The model under review builds one solid part; all positions refer to its coordinate system, in mm. Face numbers are marked on the shaded views. A direction names the side the tool comes from. Coordinates: 2 decimals unless noted, no trailing zeros. Loops run counter-clockwise (first coordinate to the right, second up) from the corner with the lowest first, then second, coordinate; pieces in that order, holes last. Notation, with made-up numbers: M 43,-27.75 L 86,-27.75 A21 cw 86,-1.75 Z; hole C -39,77.5 d1. An arc over 180 degrees is marked long. Use CSV: the item, a comma, the result in double quotes. Start each with the question number.
1. Add section A-A, the plane z = -19.5. Write out the cut boundary in (x, y), then the cut area to 3 significant figures.
2. Draft analysis for pull direction X (two halves, no side actions). For the marked faces 4, 5, 6 and 7, state which applies: +X half, -X half, draft (parallel to the pull), parting line (faces both ways), or undercut.
3. Add section B-B, the plane x = -1. Write out the cut boundary in (y, z).
4. Clearance check with flat-ended pins moving along their axes: P1, Ø1.4, axis at x = -9.48, z = -4.81, coming from the -Y side; P2, Ø7.5, axis at x = 0, z = 0, coming from the +Y side; P3, Ø4, axis at y = 7.5, z = -31, coming from the -X side; P4, Ø4, axis at x = 18.5, z = -14.5, coming from the -Y side. State where each tip first meets the part, or that it passes through.
5. For L1, parallel to X at y = 2.75, z = -12.5; L2, parallel to Z at x = 12.5, y = 5.5; L3, parallel to Y at x = -1, z = -40, list the stretches that pass through material, from the lowest coordinate up.
6. Add section D-D, the plane x = -20. Write out the cut boundary in (y, z).
7. Tool access review of the marked faces 1, 2 and 3: name each direction out of +Z, -Z, +X, -X, +Y, -Y from which nothing blocks a thin tool from reaching the whole face with its end or side.
8. Add section C-C, the plane x = 23. Write out the cut boundary in (y, z), then the cut area to 3 significant figures.
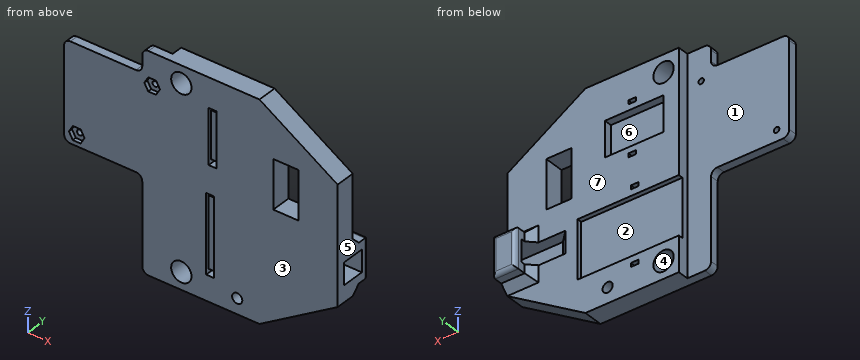
from build123d import *

# Parameters (mm, degrees)
SKETCH1_R               = 1.651
SKETCH1_R_2             = 3.302
SKETCH1_R_3             = 0.889
SKETCH1_W               = 8.2042
SKETCH1_H               = 15.748
BOSS_EXTRUDE1_DEPTH     = 6.35
SKETCH2_W               = 19.05
SKETCH2_H               = 11.43
CUT_EXTRUDE1_DEPTH      = 2.54
CUT_EXTRUDE2_DEPTH      = 83.161835082
CUT_EXTRUDE2_DEPTH_BACK = 83.161835082
SKETCH5_W               = 2.54
SKETCH5_H               = 1.27
SKETCH6_W               = 2.54
SKETCH6_H               = 15.24
CUT_EXTRUDE3_DEPTH      = 1.016
SKETCH7_W               = 40.64
SKETCH7_H               = 18.796
CUT_EXTRUDE4_DEPTH      = 1.524
CUT_EXTRUDE5_DEPTH      = 83.161835082
CUT_EXTRUDE5_DEPTH_BACK = 83.161835082
SKETCH8_W               = 2.54
SKETCH8_H               = 1.27
SKETCH10_W              = 2.54
SKETCH10_H              = 22.86
CUT_EXTRUDE6_DEPTH      = 1.016
SKETCH11_W              = 7.62
SKETCH11_H              = 12.7
BOSS_EXTRUDE2_DEPTH     = 6.35
SKETCH13_W              = 7.112
SKETCH13_H              = 7.493
CUT_EXTRUDE7_DEPTH      = 19.05
CHAMFER3_SIZE           = 2.54
FILLET1_R               = 1.27
CHAMFER4_SIZE           = 3.81
SKETCH14_W              = 33.125812981
SKETCH14_H              = 69.85
CUT_EXTRUDE8_DEPTH      = 3.556
FILLET2_R               = 2.032
CUT_EXTRUDE9_DEPTH      = 1.27


with BuildPart() as part:
    # Sketch1 → Boss-Extrude1 (new body)
    with BuildSketch(Plane(origin=(0, 0, 0), x_dir=(1, 0, 0), z_dir=(0, 1, 0))):
        Polygon((25.4, 64.262), (-12.7, 64.262), (-12.7, 33.782), (-38.1, 33.782), (-38.1, 2.032), (-12.7, 2.032), (-12.7, -5.588), (25.4, -5.588), (50.8, 10.287), (50.8, 48.387), align=None)
        with Locations(Location((18.161, 59.309, 0), (0, 0, 270))):
            Circle(SKETCH1_R, mode=Mode.SUBTRACT)
        with Locations(Location((0, 0, 0), (0, 0, 270))):
            Circle(SKETCH1_R_2, mode=Mode.SUBTRACT)
        with Locations(Location((-9.47933438, 4.811158086, 0), (0, 0, 270))):
            Circle(SKETCH1_R_3, mode=Mode.SUBTRACT)
        with Locations(Location((0, 58.674, 0), (0, 0, 270))):
            Circle(SKETCH1_R_2, mode=Mode.SUBTRACT)
        with Locations((33.9979, 18.923)):
            Rectangle(SKETCH1_W, SKETCH1_H, mode=Mode.SUBTRACT)
        with Locations(Location((-34.005247297, 30.20787503, 0), (0, 0, 270))):
            Circle(SKETCH1_R_3, mode=Mode.SUBTRACT)
    extrude(amount=BOSS_EXTRUDE1_DEPTH)

    # Sketch2 → Cut-Extrude1 (cut)
    with BuildSketch(Plane(origin=(0, 6.35, 0), x_dir=(1, 0, 0), z_dir=(0, 1, 0))):
        with Locations((9.525, 12.827)):
            Rectangle(SKETCH2_W, SKETCH2_H)
    extrude(amount=-CUT_EXTRUDE1_DEPTH, mode=Mode.SUBTRACT)

    # Sketch5 → Cut-Extrude2 (cut, two sides: drawn at the far end of the back side and taken through both)
    with BuildSketch(Plane(origin=(0, 6.35, 0), x_dir=(1, 0, 0), z_dir=(0, 1, 0)).offset(-CUT_EXTRUDE2_DEPTH_BACK)):
        with Locations((10.16, 21.082)):
            Rectangle(SKETCH5_W, SKETCH5_H)
        with Locations((10.16, 4.572)):
            Rectangle(SKETCH5_W, SKETCH5_H)
    extrude(amount=CUT_EXTRUDE2_DEPTH + CUT_EXTRUDE2_DEPTH_BACK, mode=Mode.SUBTRACT)

    # Sketch6 → Cut-Extrude3 (cut)
    with BuildSketch(Plane.XZ):
        with Locations((10.16, -12.827)):
            Rectangle(SKETCH6_W, SKETCH6_H)
    extrude(amount=-CUT_EXTRUDE3_DEPTH, mode=Mode.SUBTRACT)

    # Sketch7 → Cut-Extrude4 (cut)
    with BuildSketch(Plane(origin=(0, 6.35, 0), x_dir=(1, 0, 0), z_dir=(0, 1, 0))):
        with Locations((7.62, 43.434)):
            Rectangle(SKETCH7_W, SKETCH7_H)
    extrude(amount=-CUT_EXTRUDE4_DEPTH, mode=Mode.SUBTRACT)

    # Sketch8 → Cut-Extrude5 (cut, two sides: drawn at the far end of the back side and taken through both)
    with BuildSketch(Plane(origin=(0, 6.35, 0), x_dir=(1, 0, 0), z_dir=(0, 1, 0)).offset(-CUT_EXTRUDE5_DEPTH_BACK)):
        with Locations((9.344785272, 55.499)):
            Rectangle(SKETCH8_W, SKETCH8_H)
        with Locations((9.344785272, 31.369)):
            Rectangle(SKETCH8_W, SKETCH8_H)
    extrude(amount=CUT_EXTRUDE5_DEPTH + CUT_EXTRUDE5_DEPTH_BACK, mode=Mode.SUBTRACT)

    # Sketch10 → Cut-Extrude6 (cut)
    with BuildSketch(Plane.XZ):
        with Locations((9.344785272, -43.434)):
            Rectangle(SKETCH10_W, SKETCH10_H)
    extrude(amount=-CUT_EXTRUDE6_DEPTH, mode=Mode.SUBTRACT)

    # Sketch11 → Boss-Extrude2 (add)
    with BuildSketch(Plane(origin=(0, 6.35, 0), x_dir=(1, 0, 0), z_dir=(0, 1, 0))):
        with Locations((46.99, 39.497)):
            Rectangle(SKETCH11_W, SKETCH11_H)
    extrude(amount=BOSS_EXTRUDE2_DEPTH)

    # Sketch13 → Cut-Extrude7 (cut)
    with BuildSketch(Plane(origin=(50.8, 0, 0), x_dir=(0, 0, -1), z_dir=(1, 0, 0))):
        with Locations((39.497, 6.4135)):
            Rectangle(SKETCH13_W, SKETCH13_H)
    extrude(amount=-CUT_EXTRUDE7_DEPTH, mode=Mode.SUBTRACT)

    # Chamfer3
    chamfer3_edges = [part.edges().sort_by_distance(p)[0] for p in [
        (46.99, 6.35, -45.847),
        (43.18, 6.35, -44.45),
        (46.99, 6.35, -33.147),
        (43.18, 6.35, -34.544),
    ]]
    chamfer(chamfer3_edges, length=CHAMFER3_SIZE)

    # Fillet1
    fillet1_edges = [part.edges().sort_by_distance(p)[0] for p in [
        (50.8, 12.7, -39.497),
        (46.99, 12.7, -45.847),
        (43.18, 12.7, -39.497),
        (46.99, 12.7, -33.147),
    ]]
    fillet(fillet1_edges, radius=FILLET1_R)

    # Chamfer4
    # the kernel refuses this chamfer: 3.81 mm, written as the material it adds along each edge
    with BuildSketch(Plane(origin=(31.75, 2.667, -52.851112184), x_dir=(0.9996219169112968, -0.027495876610586386, 0), z_dir=(0, 0, 1))) as chamfer4_piece_1_section:
        Polygon((CHAMFER4_SIZE * 0.999621916911, CHAMFER4_SIZE * 0.0274958766106), (-CHAMFER4_SIZE * 0.0274958766106, CHAMFER4_SIZE * 0.999621916911), (0, 0), align=None)
    chamfer4_piece_1 = extrude(amount=26.708224368, mode=Mode.PRIVATE)
    chamfer4_piece_1 = split(chamfer4_piece_1, bisect_by=Plane(origin=(33.021365591, 6.35, -39.497), z_dir=(0, -1, 0)), keep=Keep.TOP, mode=Mode.PRIVATE)
    chamfer4_piece_1 = split(chamfer4_piece_1, bisect_by=Plane(origin=(33.021365591, 3.934268817, -26.797), z_dir=(0, 0, -1)), keep=Keep.TOP, mode=Mode.PRIVATE)
    add(chamfer4_piece_1)

    # Sketch14 → Cut-Extrude8 (cut)
    with BuildSketch(Plane(origin=(0, 6.35, 0), x_dir=(1, 0, 0), z_dir=(0, 1, 0))):
        with Locations((-21.53709351, 29.337)):
            Rectangle(SKETCH14_W, SKETCH14_H)
    extrude(amount=-CUT_EXTRUDE8_DEPTH, mode=Mode.SUBTRACT)

    # Fillet2
    fillet2_edges = [part.edges().sort_by_distance(p)[0] for p in [
        (-38.1, 1.397, -33.782),
        (-12.7, 1.397, -33.782),
        (-12.7, 1.397, -2.032),
        (-38.1, 1.397, -2.032),
        (-12.7, 1.397, -64.262),
        (-12.7, 1.397, 5.588),
    ]]
    fillet(fillet2_edges, radius=FILLET2_R)

    # Sketch16 → Cut-Extrude9 (cut)
    with BuildSketch(Plane.XZ):
        Polygon((-10.74933438, -7.010862612), (-8.20933438, -7.010862612), (-6.93933438, -4.811158086), (-8.20933438, -2.61145356), (-10.74933438, -2.61145356), (-12.01933438, -4.811158086), align=None)
        Polygon((-32.74988098, -32.415963663), (-31.465303289, -30.224740225), (-32.720669607, -28.016651592), (-35.260613615, -27.999786398), (-36.545191306, -30.191009836), (-35.289824988, -32.399098469), align=None)
    extrude(amount=-CUT_EXTRUDE9_DEPTH, mode=Mode.SUBTRACT)


solid = part.part
Computed:
1,outline,"M -38.1,0 L 8.89,0 L 8.89,1.02 L 11.43,1.02 L 11.43,0 L 29.9,0 L 29.9,6.35 L -4.97,6.35 L -4.97,2.79 L -38.1,2.79 Z; M 38.1,0 L 50.8,0 L 50.8,6.35 L 38.1,6.35 Z"
1,area,"392 mm^2"
2,face 4,"undercut"
2,face 5,"+X half"
2,face 6,"undercut"
2,face 7,"draft"
3,outline,"M 0,-64.26 L 6.35,-64.26 L 6.35,-61.82 L 0,-61.82 Z; M 0,-55.53 L 6.35,-55.53 L 6.35,-52.83 L 4.83,-52.83 L 4.83,-34.04 L 6.35,-34.04 L 6.35,-3.15 L 0,-3.15 Z; M 0,3.15 L 6.35,3.15 L 6.35,5.59 L 0,5.59 Z"
4,P1,"passes through"
4,P2,"stops at y = 6.35"
4,P3,"stops at x = -4.97"
4,P4,"stops at y = 0"
5,L1,"x = -38.1 to 29.9, 38.1 to 50.8"
5,L2,"z = -64.26 to -52.83, -34.04 to -18.54, -7.11 to 5.59"
5,L3,"y = 0 to 4.83"
6,outline,"M 0,-33.78 L 2.79,-33.78 L 2.79,-2.03 L 0,-2.03 Z"
7,face 1,"+Z, -Z, -X, +Y"
7,face 2,"-X, +Y"
7,face 3,"+Z, -Z, +X, -X, -Y"
8,outline,"M 0,-64.26 L 6.35,-64.26 L 6.35,-52.83 L 4.83,-52.83 L 4.83,-34.04 L 6.35,-34.04 L 6.35,5.59 L 0,5.59 Z"
8,area,"415 mm^2"
